Autodesk Inventor part; units mm, degrees
ref_plane "YZ Plane" through (0, 0, 0) normal (1, 0, 0) x (0, 1, 0)
ref_plane "XZ Plane" through (0, 0, 0) normal (0, 1, 0) x (-1, 0, 0)
ref_plane "XY Plane" through (0, 0, 0) normal (0, 0, 1) x (1, 0, 0)
sketch "Szkic1" plane through (0, 0, 0) normal (0, 1, 0) x (-1, 0, 0)
  line L0 (-25.25, -37.75) -> (25.25, -37.75)
  line L1 (25.25, -37.75) -> (25.25, 37.75)
  line L2 (25.25, 37.75) -> (-25.25, 37.75)
  line L3 (-25.25, 37.75) -> (-25.25, -37.75)
  line L4 (-25.25, -37.75) -> (25.25, 37.75) construction
  line L5 (25.25, -37.75) -> (-25.25, 37.75) construction
  point P0 (0, 0)
  dimension "d0" = 50.5
  dimension "d1" = 75.5
extrude "Wyciągnięcie proste1" add sketch "Szkic1" along normal blind 2
sketch "Szkic2" plane through (0, 2, 0) normal (0, 1, 0) x (1, 0, 0)
  line L0 (25.25, 37.75) -> (-25.25, 37.75)
  line L1 (-25.25, 37.75) -> (-25.25, -37.75)
  line L2 (-25.25, -37.75) -> (25.25, -37.75)
  line L3 (25.25, -37.75) -> (25.25, 37.75)
  line L4 (-25.25, 37.75) -> (-25.25, -37.75)
  point P0 (0, 0)
  point P1 (-21.5, -34.5)
  point P2 (-21.5, 34.5)
  point P3 (21.5, 34.5)
  point P4 (21.5, -34.5)
  point P5 (-15.25, 14.5)
  point P6 (15.25, 14.5)
  dimension "d4" = 69
  dimension "d5" = 69
  dimension "d6" = 43
  dimension "d7" = 43
  dimension "d8" = 75.5
  dimension "d9" = 50.5
  dimension "d10" = 3.75
  dimension "d11" = 3.25
  dimension "d13" = 3.75
  dimension "d14" = 3.25
  dimension "d15" = 20
  dimension "d16" = 20
  dimension "d17" = 30.5
  dimension "d19" = 10
  dimension "d20" = 10
hole "Otwór1" at (-21.5, 2, 34.5) at (-21.5, 2, -34.5) at (21.5, 2, -34.5) at (21.5, 2, 34.5) at (-15.25, 2, -14.5) at (15.25, 2, -14.5) direction (0, -1, 0) diameter 3.5 end through all
sketch "Szkic3" plane through (0, 2, 0) normal (0, 1, 0) x (1, 0, 0)
  circle A0 centre (-15.25, 14.5) radius 1.75
  circle A1 centre (21.5, 34.5) radius 1.75
  circle A2 centre (-21.5, -34.5) radius 1.75
  circle A3 centre (-21.5, 34.5) radius 1.75
  circle A4 centre (21.5, -34.5) radius 1.75
  circle A5 centre (15.25, 14.5) radius 1.75
  line L0 (25.25, 37.75) -> (-25.25, 37.75)
  line L1 (-25.25, 37.75) -> (-25.25, -37.75)
  line L2 (-25.25, -37.75) -> (25.25, -37.75)
  line L3 (25.25, -37.75) -> (25.25, 37.75)
  line L4 (-15.25, 37.75) -> (15.25, 37.75)
  line L5 (15.25, 37.75) -> (15.25, 27.25)
  line L6 (15.25, 27.25) -> (-15.25, 27.25)
  line L7 (-15.25, 27.25) -> (-15.25, 37.75)
  circle A6 centre (20.8161, 25.0959) radius 5
  line L8 (-15.25, -37.75) -> (15.25, -37.75)
  line L9 (15.25, -37.75) -> (15.25, -27.25)
  line L10 (15.25, -27.25) -> (-15.25, -27.25)
  line L11 (-15.25, -27.25) -> (-15.25, -37.75)
  line L12 (-25.25, -27.25) -> (-15.25, -27.25)
  line L13 (-15.25, -27.25) -> (-15.25, 7.75)
  line L14 (-15.25, 7.75) -> (-25.25, 7.75)
  line L15 (-25.25, 7.75) -> (-25.25, -27.25)
  circle A7 centre (20.8161, -3.2547) radius 3
  point P0 (0, 0)
  dimension "d28" = 10.5
  dimension "d29" = 10
  dimension "d30" = 10
  dimension "d31" = 10
  dimension "d32" = 10.5
  dimension "d33" = 10
  dimension "d34" = 10
  dimension "d35" = 35
  dimension "d36" = 6
extrude "Wyciągnięcie proste2" add sketch "Szkic3" along normal blind 18 contours L5 L6 L7 L0 | A6 L3 | L3 A6 | L2 L11 L10 L9 | A7
sketch "Szkic4" plane through (0, 2, 0) normal (0, 1, 0) x (1, 0, 0)
  line L0 (15.25, -27.25) -> (15.25, -37.75)
  line L1 (15.25, -37.75) -> (25.25, -37.75)
  line L2 (25.25, -37.75) -> (25.25, 22.7849)
  arc A0 (25.25, 27.4069) -> (25.25, 22.7849) centre (20.8161, 25.0959) ccw
  line L3 (25.25, 27.4069) -> (25.25, 37.75)
  line L4 (25.25, 37.75) -> (15.25, 37.75)
  line L5 (15.25, 37.75) -> (15.25, 27.25)
  line L6 (15.25, 27.25) -> (-15.25, 27.25)
  line L7 (-15.25, 27.25) -> (-15.25, 37.75)
  line L8 (-15.25, 37.75) -> (-25.25, 37.75)
  line L9 (-25.25, 37.75) -> (-25.25, -37.75)
  line L10 (-25.25, -37.75) -> (-15.25, -37.75)
  line L11 (-15.25, -37.75) -> (-15.25, -27.25)
  line L12 (-15.25, -27.25) -> (15.25, -27.25)
  circle A1 centre (20.8161, -3.2547) radius 3
  circle A2 centre (-15.25, 14.5) radius 1.75
  circle A3 centre (21.5, 34.5) radius 1.75
  circle A4 centre (-21.5, -34.5) radius 1.75
  circle A5 centre (-21.5, 34.5) radius 1.75
  circle A6 centre (21.5, -34.5) radius 1.75
  circle A7 centre (15.25, 14.5) radius 1.75
  line L13 (-25.25, 37.75) -> (-25.25, -37.75)
  line L14 (-25.25, -27.25) -> (-14.25, -27.25)
  line L15 (-14.25, -27.25) -> (-14.25, 7.75)
  line L16 (-14.25, 7.75) -> (-25.25, 7.75)
  line L17 (-25.25, 7.75) -> (-25.25, -27.25)
  point P0 (0, 0)
  dimension "d39" = 11
  dimension "d40" = 35
extrude "Wyciągnięcie proste3" add sketch "Szkic4" along normal blind 6 contours L12 L14 L9 L16 L15
sketch "Szkic5" plane through (0, 0, 0) normal (0, -1, 0) x (1, 0, 0)
  circle A0 centre (-15.25, -14.5) radius 1.75
  circle A1 centre (21.5, -34.5) radius 1.75
  circle A2 centre (-21.5, 34.5) radius 1.75
  circle A3 centre (-21.5, -34.5) radius 1.75
  circle A4 centre (21.5, 34.5) radius 1.75
  circle A5 centre (15.25, -14.5) radius 1.75
  line L0 (25.25, -37.75) -> (-25.25, -37.75)
  line L1 (25.25, 37.75) -> (25.25, -37.75)
  line L2 (-25.25, 37.75) -> (25.25, 37.75)
  line L3 (-25.25, -37.75) -> (-25.25, 37.75)
  line L4 (-18, -7.5) -> (18, -7.5)
  line L5 (18, -21.5) -> (-18, -21.5)
  arc A6 (-15.25, -17.25) -> (-15.25, -11.75) centre (-15.25, -14.5) ccw
  arc A7 (15.25, -11.75) -> (15.25, -17.25) centre (15.25, -14.5) ccw
  line L6 (-15.25, -11.75) -> (-18, -11.75)
  line L7 (-15.25, -17.25) -> (-18, -17.25)
  line L8 (15.25, -11.75) -> (18, -11.75)
  line L9 (15.25, -17.25) -> (18, -17.25)
  line L10 (-18, -21.5) -> (-18, -17.25)
  line L11 (-18, -11.75) -> (-18, -7.5)
  line L12 (18, -7.5) -> (18, -11.75)
  line L13 (18, -17.25) -> (18, -21.5)
  point P0 (0, 0)
  dimension "d43" = 36
  dimension "d44" = 14
  dimension "d45" = 7
  dimension "d46" = 7
extrude "Wyciągnięcie proste4" add sketch "Szkic5" along normal blind 5 contours L4 L12 L8 A7 L9 L13 L5 L10 L7 A6 L6 L11
equation "\"d30\" = d29"
equation "\"d34\" = d33"
equation "\"d45\" = d46"
equation "\"d47\" = d48"
properties part number "step driver"
The model under review builds one solid part; all positions refer to its coordinate system, in mm. A direction names the side the tool comes from. Round coordinates to 2 decimals unless told otherwise and drop trailing zeros. Order: outer loops, then holes, each group sorted by start corner. A loop starts at its lowest first (then second) coordinate and runs counter-clockwise, first axis right, second up. Notation, with made-up numbers: (12, -15.75) -> (27, -15.75) arc R31 cw to (27, 10.25) -> close; hole circle Ø6 at (29, 22). An arc over 180 degrees is marked (long way). Use a Markdown table: item, result.
Q1. Tool access review of faces 4 (the flat face through (-18, -2, -10)), 5 (the flat face through (18, -2, -19)), 6 (the flat face through (17, -2, -17.25)): name each direction out of +Z, -Z, +X, -X, +Y, -Y from which nothing blocks a thin tool from reaching the whole face with its end or side.
Values:
| item | result |
|---|---|
| face 4 | +Z, -Z, -X, -Y |
| face 5 | +Z, -Z, +X, -Y |
| face 6 | +X, -Y |
Q2. We need section A-A on x = -21.5. Write out the cut boundary in (y, z).
Values:
| item | result |
|---|---|
| outline | (0, -37.75) -> (2, -37.75) -> (2, -36.25) -> (0, -36.25) -> close; (0, -32.75) -> (2, -32.75) -> (2, -7.75) -> (8, -7.75) -> (8, 27.25) -> (2, 27.25) -> (2, 32.75) -> (0, 32.75) -> close; (0, 36.25) -> (2, 36.25) -> (2, 37.75) -> (0, 37.75) -> close |
Q3. Clearance check with flat-ended pins moving along their axes: P1, Ø8, axis at x = -18.5, z = 17.5, coming from the +Y side; P2, Ø15, axis at x = 3.5, z = 1.5, coming from the -Y side; P3, Ø2, axis at x = 21.5, z = -34.5, coming from the -Y side; P4, Ø1.8, axis at x = -19, y = 6.5, coming from the -Z side. State where each tip first meets the part, or that it passes through.
Values:
| item | result |
|---|---|
| P1 | stops at y = 8 |
| P2 | stops at y = 0 |
| P3 | passes through |
| P4 | stops at z = -7.75 |
Q4. We need section C-C on x = 10. Write out the cut boundary in (y, z), then the cut area to 3 significant figures.
Values:
| item | result |
|---|---|
| outline | (-5, -21.5) -> (0, -21.5) -> (0, -37.75) -> (20, -37.75) -> (20, -27.25) -> (2, -27.25) -> (2, 27.25) -> (20, 27.25) -> (20, 37.75) -> (0, 37.75) -> (0, -7.5) -> (-5, -7.5) -> close |
| area | 599 mm^2 |
Q5. We need section B-B on z = -14.5. Write out the cut boundary in (x, y), then the cut area to 3 significant figures.
Values:
| item | result |
|---|---|
| outline | (-25.25, 0) -> (-17, 0) -> (-17, 2) -> (-25.25, 2) -> close; (-13.5, 0) -> (-12.5, 0) -> (-12.5, -5) -> (12.5, -5) -> (12.5, 0) -> (13.5, 0) -> (13.5, 2) -> (-13.5, 2) -> close; (17, 0) -> (25.25, 0) -> (25.25, 2) -> (17, 2) -> close |
| area | 212 mm^2 |
Q6. We need section D-D on y = -1. Write out the cut boundary in (x, z).
Values:
| item | result |
|---|---|
| outline | (-18, -21.5) -> (18, -21.5) -> (18, -17.25) -> (15.25, -17.25) arc R2.75 cw to (15.25, -11.75) -> (18, -11.75) -> (18, -7.5) -> (-18, -7.5) -> (-18, -11.75) -> (-15.25, -11.75) arc R2.75 cw to (-15.25, -17.25) -> (-18, -17.25) -> close |
Q7. For line 1 (X direction, y = 1.05, z = 34.5); line 2 (Z direction, x = -21.5, y = 1.5); line 3 (Z direction, x = 13, y = 8.75), list the stretches that pass through material, from the lowest coordinate up.
Values:
| item | result |
|---|---|
| line 1 | x = -25.25 to -23.25, -19.75 to 19.75, 23.25 to 25.25 |
| line 2 | z = -37.75 to -36.25, -32.75 to 32.75, 36.25 to 37.75 |
| line 3 | z = -37.75 to -27.25, 27.25 to 37.75 |
Q8. Mouldability with a two-part tool opening along X and no side actions: class faces 1 (the cylindrical face through (-16.726, 0.986, -13.559)), 2 (the flat face through (21, 20, -25)), 3 (the cylindrical face through (12.5, -2.5, -14.6)) as +X half, -X half, draft (parallel to the pull), parting line (faces both ways), or undercut.
Values:
| item | result |
|---|---|
| face 1 | undercut |
| face 2 | draft |
| face 3 | +X half |
